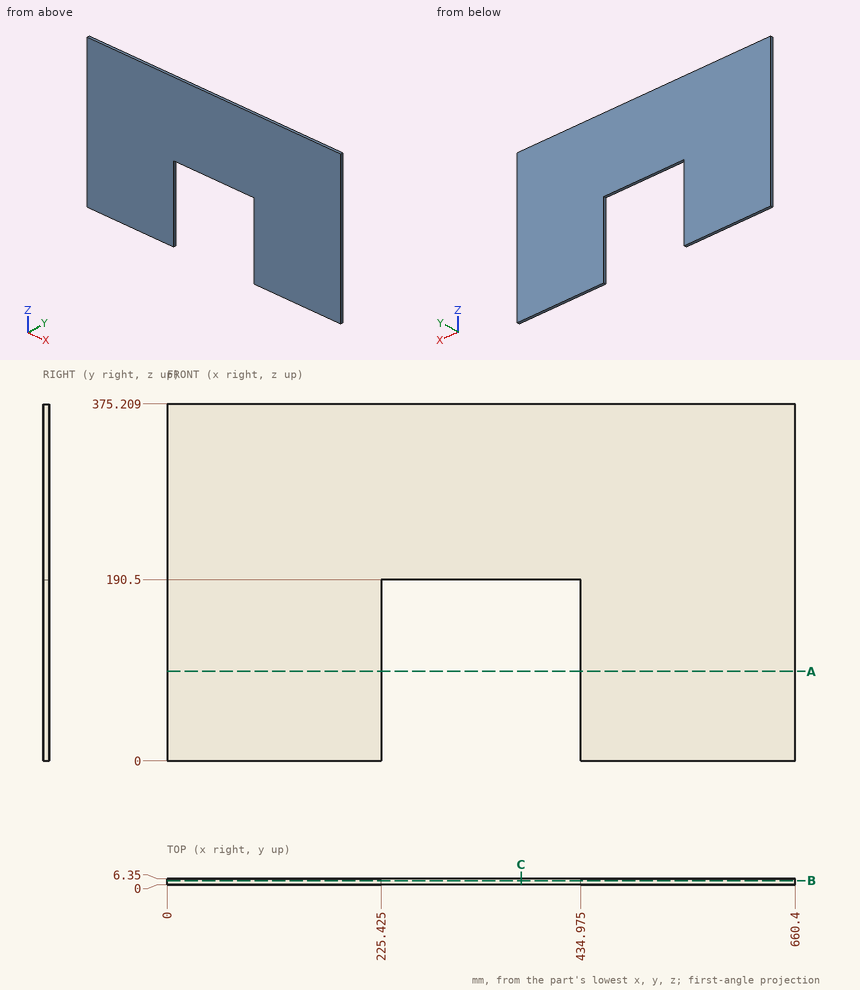
Drawing for the job (mm, zero at the part's lowest x, y, z). Round coordinates to 2 decimals unless told otherwise and drop trailing zeros. Order: outer loops, then holes, each group sorted by start corner. A loop starts at its lowest first (then second) coordinate and runs counter-clockwise, first axis right, second up. Notation, with made-up numbers: (-26.75, -6) -> (-22.75, -6) arc R28 ccw to (-22.75, 20) -> close; hole circle Ø2 at (76, 50). An arc over 180 degrees is marked (long way). Put each result on its own line as item: value.
Q1. Band-saw the part on C-C (x = 372.5). Give the cut face in (y, z).
From the geometry:
outline: (0, 190.5) -> (6.35, 190.5) -> (6.35, 375.21) -> (0, 375.21) -> close
Q2. Band-saw the part on A-A (z = 94). Give the cut face in (x, y) (3 decimals).
From the geometry:
outline: (0, 0) -> (225.425, 0) -> (225.425, 6.35) -> (0, 6.35) -> close; (434.975, 0) -> (660.4, 0) -> (660.4, 6.35) -> (434.975, 6.35) -> close
Q3. Pin check, flat tip, straight feed: pin 1 Ø3 at (x, y) = (363.5, 1.5) entering from -Z. Stop position of the tip, or through.
From the geometry:
pin 1: stops at z = 190.5
Q4. Band-saw the part on B-B (y = 4.5). Give the cut face in (x, z) (1 decimal), and give its area (3 significant figures).
From the geometry:
outline: (0, 0) -> (225.4, 0) -> (225.4, 190.5) -> (435, 190.5) -> (435, 0) -> (660.4, 0) -> (660.4, 375.2) -> (0, 375.2) -> close
area: 208,000 mm2
Q5. Wall check: line 1 (X direction, y = 5.25, z = 41.5) (3 decimals); line 2 (Z direction, x = 326, y = 1.5). Give the ranges that are in metal, low to high. Write a range as [from, to].
From the geometry:
line 1: x = [0, 225.425], [434.975, 660.4]
line 2: z = [190.5, 375.21]
